```python
from build123d import *

# Parameters (mm, degrees)
SKETCH1_W           = 3
SKETCH1_H           = 12
BOSS_EXTRUDE1_DEPTH = 20
SKETCH2_R           = 5
CUT_EXTRUDE1_DEPTH  = 19
SKETCH6_W           = 3
SKETCH6_H           = 12
BOSS_EXTRUDE3_DEPTH = 12
SKETCH13_W          = 1.8
SKETCH13_H          = 12
BOSS_EXTRUDE4_DEPTH = 1
SKETCH7_R           = 2
CUT_EXTRUDE2_DEPTH  = 10
CUT_EXTRUDE3_DEPTH  = 1
SKETCH11_R          = 1.6
CUT_EXTRUDE4_DEPTH  = 0.6
SKETCH12_R          = 0.9
CUT_EXTRUDE5_DEPTH  = 24.446961424
FILLET2_R           = 1


with BuildPart() as part:
    # Sketch1 → Boss-Extrude1 (new body)
    with BuildSketch(Plane.XY):
        with Locations((1.5, 6)):
            Rectangle(SKETCH1_W, SKETCH1_H)
    extrude(amount=-BOSS_EXTRUDE1_DEPTH)

    # Sketch2 → Cut-Extrude1 (cut)
    with BuildSketch(Plane.XY):
        with Locations((3, 6)):
            Circle(SKETCH2_R)
    extrude(amount=-CUT_EXTRUDE1_DEPTH, mode=Mode.SUBTRACT)

    # Sketch6 → Boss-Extrude3 (add)
    with BuildSketch(Plane.XY):
        with Locations((1.5, 6)):
            Rectangle(SKETCH6_W, SKETCH6_H)
    extrude(amount=BOSS_EXTRUDE3_DEPTH)

    # Sketch13 → Boss-Extrude4 (add)
    with BuildSketch(Plane.XY):
        with Locations((0.9, 6)):
            Rectangle(SKETCH13_W, SKETCH13_H)
    extrude(amount=-BOSS_EXTRUDE4_DEPTH)

    # Sketch7 → Cut-Extrude2 (cut)
    with BuildSketch(Plane(origin=(0, 0, 0), x_dir=(-1, 0, 0), z_dir=(0, 0, -1))):
        with Locations((-3, 6)):
            Circle(SKETCH7_R)
    extrude(amount=-CUT_EXTRUDE2_DEPTH, mode=Mode.SUBTRACT)

    # Sketch10 → Cut-Extrude3 (cut)
    with BuildSketch(Plane(origin=(0, 0, 10), x_dir=(-1, 0, 0), z_dir=(0, 0, -1))):
        with BuildLine():
            Line((-3, 7), (-1.267949192, 7))
            ThreePointArc((-1.267949192, 7), (-1, 6), (-1.267949192, 5))
            Line((-1.267949192, 5), (-3, 5))
            Line((-3, 5), (-3, 7))
        make_face()
    extrude(amount=-CUT_EXTRUDE3_DEPTH, mode=Mode.SUBTRACT)

    # Sketch11 → Cut-Extrude4 (cut)
    with BuildSketch(Plane.ZY):
        with Locations((6, 9.5)):
            Circle(SKETCH11_R)
    cut_extrude4 = extrude(amount=-CUT_EXTRUDE4_DEPTH, mode=Mode.SUBTRACT)

    # Sketch12 → Cut-Extrude5 (cut, through all)
    with BuildSketch(Plane.ZY.offset(-0.6)):
        with Locations((6, 9.5)):
            Circle(SKETCH12_R)
    cut_extrude5 = extrude(amount=-CUT_EXTRUDE5_DEPTH, mode=Mode.SUBTRACT)

    # Mirror1: Cut-Extrude4, Cut-Extrude5 across plane
    add(cut_extrude4.mirror(Plane(origin=(0, 6, 0), x_dir=(0, 0, 1), z_dir=(0, -1, 0))), mode=Mode.SUBTRACT)
    add(cut_extrude5.mirror(Plane(origin=(0, 6, 0), x_dir=(0, 0, 1), z_dir=(0, -1, 0))), mode=Mode.SUBTRACT)

    # Fillet2
    fillet2_edges = [part.edges().sort_by_distance(p)[0] for p in [
        (1.5, 0, -20),
        (1.5, 12, 12),
        (1.5, 0, 12),
        (1.5, 12, -20),
    ]]
    fillet(fillet2_edges, radius=FILLET2_R)

    # Sketch16 → Revolve3 (revolve)
    with BuildSketch(Plane(origin=(0, 0, -19.4), x_dir=(-1, 0, 0), z_dir=(0, 0, -1)), mode=Mode.PRIVATE) as revolve3_sk:
        with BuildLine():
            Line((-3.25, 11.4), (-3, 11.4))
            Line((-3, 11.4), (-3, 11.15))
            ThreePointArc((-3, 11.15), (-3.176776695, 11.223223305), (-3.25, 11.4))
        make_face()
    revolve3 = revolve(revolve3_sk.sketch.rotate(Axis((3.25, 11.4, -19.4), (-1, 0, 0)), 180), axis=Axis((3.25, 11.4, -19.4), (-1, 0, 0)))

    # Mirror2: Revolve3 across plane
    add(revolve3.mirror(Plane(origin=(0, 6, 0), x_dir=(0, 0, 1), z_dir=(0, -1, 0))))

    # Mirror2 at the second plane: Revolve3 across plane
    add(revolve3.mirror(Plane.XY.offset(-4)))

    # Mirror2 at the second plane copy 1 sketc → Mirror2 at the second plane copy 1 (revolve)
    with BuildSketch(Plane(origin=(0, 12, 11.4), x_dir=(-1, 0, 0), z_dir=(0, 0, 1))):
        with BuildLine():
            Line((-3.25, 11.4), (-3, 11.4))
            Line((-3, 11.4), (-3, 11.15))
            ThreePointArc((-3, 11.15), (-3.176776695, 11.223223305), (-3.25, 11.4))
        make_face()
    revolve(axis=Axis((3.25, 0.6, 11.4), (-1, 0, 0)))


solid = part.part
```
Input: part model. Units: mm. Frame: model coordinates. A direction names the side the tool comes from. Give positions to 0.01 mm unless a question says otherwise; leave off trailing zeros. Order: outer loops, then holes, each group sorted by start corner. A loop starts at its lowest first (then second) coordinate and runs counter-clockwise, first axis right, second up. Notation, with made-up numbers: M -8.75,70.25 L 31.25,70.25 A20 ccw 31.25,102.25 Z; hole C -12,-11.5 d5. An arc over 180 degrees is marked long. Return JSON: item names as keys, results as strings.
1) Line query: L1, parallel to Z at x = 2.1, y = 2.5; L2, parallel to Y at x = 0.55, z = 6; L3, parallel to Z at x = 0.35, y = 2.5. Output: solid intervals per line, ascending. Write a range as [from, to].
Taken from the geometry:
{"L1": "z = [-20, -19], [0, 5.1], [6.9, 12]", "L2": "y = [0, 0.9], [4.1, 7.9], [11.1, 12]", "L3": "z = [-20, -19], [-1, 4.4], [7.6, 12]"}
2) Access query for faces 4 (the face through (2.3, 7.4, 10)), 5 (the face through (1.8, 2.5, 5.1)), 6 (the face through (0.3, 3.11, 7.48)). Directions: +Z, -Z, +X, -X, +Y, -Y. A direction counts if a zero-diameter tool reaches every point of the face in a straight line with its end or side. Return the directions, or none.
Taken from the geometry:
{"face 4": "+X", "face 5": "+X, -X", "face 6": "-X"}
3) Section query B-B on y = 2.5. Output: boundary loops of the cut face in (x, z), and give its area (3 significant figures).
Taken from the geometry:
{"outline": "M 0,-20 L 3,-20 L 3,-19 L 0,-19 Z; M 0,-1 L 1.8,-1 L 1.8,0 L 3,0 L 3,5.1 L 0.6,5.1 L 0.6,4.4 L 0,4.4 Z; M 0,7.6 L 0.6,7.6 L 0.6,6.9 L 3,6.9 L 3,12 L 0,12 Z", "area": "34.6 mm2"}
4) Section query C-C on z = 6. Output: boundary loops of the cut face in (x, y).
Taken from the geometry:
{"outline": "M 0,0 L 3,0 L 3,1.6 L 0.6,1.6 L 0.6,0.9 L 0,0.9 Z; M 0,4.1 L 0.6,4.1 L 0.6,3.4 L 3,3.4 L 3,4 A2 cw 3,8 L 3,8.6 L 0.6,8.6 L 0.6,7.9 L 0,7.9 Z; M 0,11.1 L 0.6,11.1 L 0.6,10.4 L 3,10.4 L 3,12 L 0,12 Z"}
5) Section query D-D on x = 2.4. Output: boundary loops of the cut face in (y, z), and give its area (3 significant figures).
Taken from the geometry:
{"outline": "M 0,-19 A1 ccw 1,-20 L 11,-20 A1 ccw 12,-19 L 12,11 A1 ccw 11,12 L 1,12 A1 ccw 0,11 Z; hole M 1.04,-19 L 10.96,-19 L 10.96,0 L 7.91,0 L 7.91,10 L 7,10 L 7,11 L 5,11 L 5,10 L 4.09,10 L 4.09,0 L 1.04,0 Z; hole C 2.5,6 d1.8; hole C 9.5,6 d1.8", "area": "149 mm2"}
6) Section query A-A on y = 6. Output: boundary loops of the cut face in (x, z).
Taken from the geometry:
{"outline": "M 0,-20 L 3,-20 L 3,-19 L 0,-19 Z; M 0,-1 L 1.8,-1 L 1.8,0 L 1,0 L 1,11 L 3,11 L 3,12 L 0,12 Z"}
7) Contact query for flat-ended pins moving along their axis: pin 1 (6 mm diameter, centred on y = 5, z = 8.5, fed in from -X); pin 2 (3 mm diameter, centred on y = 2.5, z = 6, fed in from +X). Output: stop coordinate, or through.
Taken from the geometry:
{"pin 1": "stops at x = 0", "pin 2": "stops at x = 3"}
8) Mould query, pull axis Y, two halves, no side actions, for faces 1 (the face through (1.44, 10.75, -9.37)), 2 (the face through (1, 0, -4)), 3 (the face through (1, 6, 12)). Classes: released by +Y, released by -Y, zero draft, split by the parting line, or undercut.
Taken from the geometry:
{"face 1": "undercut", "face 2": "released by -Y", "face 3": "zero draft"}
